from build123d import *

# Parameters (mm, degrees)
BOX001_W       = 7
BOX001_H       = 2.8
BOX001_DEPTH   = 3.5
FILLET001_R    = 1
CYLINDER_R     = 1.4
CYLINDER_DEPTH = 1
BOX_W          = 6.5
BOX_H          = 2.3
BOX_DEPTH      = 6
FILLET_R       = 1


with BuildPart() as fillet001:
    # Box001 → Box001 (new body)
    with BuildSketch(Plane(origin=(-0.25, -0.25, -2), x_dir=(1, 0, 0), z_dir=(0, 0, 1))):
        with Locations((3.5, 1.4)):
            Rectangle(BOX001_W, BOX001_H)
    extrude(amount=BOX001_DEPTH)

    # Fillet001
    fillet001_edges = [fillet001.edges().sort_by_distance(p)[0] for p in [
        (-0.25, -0.25, -0.25),
        (-0.25, 2.55, -0.25),
        (6.75, -0.25, -0.25),
        (6.75, 2.55, -0.25),
    ]]
    fillet(fillet001_edges, radius=FILLET001_R)


with BuildPart() as cylinder:
    # Cylinder → Cylinder (new body)
    with BuildSketch(Plane(origin=(3.25, 1.15, -3), x_dir=(1, 0, 0), z_dir=(0, 0, 1))):
        Circle(CYLINDER_R)
    extrude(amount=CYLINDER_DEPTH)


with BuildPart() as fusion:
    # Box → Box (new body)
    with BuildSketch(Plane.XY):
        with Locations((3.25, 1.15)):
            Rectangle(BOX_W, BOX_H)
    extrude(amount=BOX_DEPTH)

    # Fillet
    fillet_edges = [fusion.edges().sort_by_distance(p)[0] for p in [
        (0, 0, 3),
        (0, 1.15, 6),
        (0, 2.3, 3),
        (6.5, 0, 3),
        (6.5, 1.15, 6),
        (6.5, 2.3, 3),
        (3.25, 0, 6),
        (3.25, 2.3, 6),
    ]]
    fillet(fillet_edges, radius=FILLET_R)

    # Fusion: union Fillet001, Cylinder
    add(fillet001.part)
    add(cylinder.part)


solid = fusion.part
For this review, take the finished solid that the model builds, in its own axes (mm). A direction names the side the tool comes from. Round coordinates to 2 decimals unless told otherwise and drop trailing zeros. Order: outer loops, then holes, each group sorted by start corner. A loop starts at its lowest first (then second) coordinate and runs counter-clockwise, first axis right, second up. Notation, with made-up numbers: M 59,81.5 L 112,81.5 A27 cw 112,103.5 Z; hole C 9.25,40.5 d4. An arc over 180 degrees is marked long. Write each question's results on one line, items separated by ' | '. Start each with the question number.
1. Tool access review of faces 1 (the face through (0.285, 1.999, 3.274)), 2 (the face through (0.285, 0.301, 3.274)), 3 (the face through (3, 2.3, 3)): name each direction out of +Z, -Z, +X, -X, +Y, -Y from which nothing blocks a thin tool from reaching the whole face with its end or side.
2. To check wall thickness, follow L1, parallel to Y at x = 2.75, z = 2.5; L2, parallel to Z at x = 6.25, y = 0.85; L3, parallel to Y at x = 6.5, z = -0.75. State the ranges of each line that lie inside material, in increasing order. Write a range as [from, to].
3. Add section B-B (y = 1.15). State the section outline as (x, z) points.
4. Add section D-D (z = 3.5). State the section outline as (x, y) points.
5. Clearance check with flat-ended pins moving along their axes: pin 1 Ø1 at (x, z) = (3, 3.5) entering from +Y; pin 2 Ø1 at (x, z) = (3.5, 3.5) entering from -Y; pin 3 Ø0.8 at (x, y) = (5.5, 0.5) entering from -Z. State where each tip first meets the part, or that it passes through.
6. Add section C-C (x = 2.75). State the section outline as (y, z) points.
7. Add section A-A (z = 0.5). State the section outline as (x, y) points.
Output values:
1) face 1: +Z, -X, +Y | face 2: +Z, -X, -Y | face 3: +Z, +X, -X, +Y
2) L1: [0, 2.3] | L2: [-2, 5.64] | L3: [0.09, 2.21]
3) outline: M -0.25,-2 L 1.85,-2 L 1.85,-3 L 4.65,-3 L 4.65,-2 L 6.75,-2 L 6.75,1.5 L 6.5,1.5 L 6.5,5 A1 ccw 5.5,6 L 1,6 A1 ccw 0,5 L 0,1.5 L -0.25,1.5 Z
4) outline: M 0,1 A1 ccw 1,0 L 5.5,0 A1 ccw 6.5,1 L 6.5,1.3 A1 ccw 5.5,2.3 L 1,2.3 A1 ccw 0,1.3 Z
5) pin 1: y = 2.3 | pin 2: y = 0 | pin 3: z = -2
6) outline: M -0.25,-2 L -0.16,-2 L -0.16,-3 L 2.46,-3 L 2.46,-2 L 2.55,-2 L 2.55,1.5 L 2.3,1.5 L 2.3,5 A1 ccw 1.3,6 L 1,6 A1 ccw 0,5 L 0,1.5 L -0.25,1.5 Z
7) outline: M -0.25,0.75 A1 ccw 0.75,-0.25 L 5.75,-0.25 A1 ccw 6.75,0.75 L 6.75,1.55 A1 ccw 5.75,2.55 L 0.75,2.55 A1 ccw -0.25,1.55 Z
